from build123d import *

# Parameters (mm, degrees)
CUT_EXTRUDE1_DEPTH                   = 8
M6_CLEARANCE_HOLE1_D                 = 7
M6_CLEARANCE_HOLE1_DEPTH             = 14
M6_CLEARANCE_HOLE1_CSINK_D           = 7.05
M6_CLEARANCE_HOLE1_CSINK_ANGLE       = 90
CIRPATTERN1_COUNT                    = 4
F_6_1_6_1_DIAMETER_HOLE1_D           = 6.1
F_6_1_6_1_DIAMETER_HOLE1_DEPTH       = 14
F_6_1_6_1_DIAMETER_HOLE1_CSINK_D     = 6.15
F_6_1_6_1_DIAMETER_HOLE1_CSINK_ANGLE = 90


with BuildPart() as part:
    # Sketch1 → Revolve1 (revolve)
    with BuildSketch(Plane.XY):
        Polygon((-14, 1), (-14, 15), (-36, 15), (-36, 13), (-38, 13), (-38, 15), (-40, 15), (-40, 4), (-49, 4), (-49, 0), (-47, 0), (-47, 2), (-45, 2), (-45, 0), (-43, 0), (-43, 1), align=None)
    revolve(axis=Axis((0, 0, 0), (0, 1, 0)))

    # Sketch2 → Cut-Extrude1 (cut)
    with BuildSketch(Plane(origin=(0, 15, 0), x_dir=(1, 0, 0), z_dir=(0, 1, 0))):
        with BuildLine():
            Line((0, 3), (29, 3))
            ThreePointArc((29, 3), (32, 0), (29, -3))
            Line((29, -3), (0, -3))
            ThreePointArc((0, -3), (-3, 0), (0, 3))
        make_face()
    extrude(amount=-CUT_EXTRUDE1_DEPTH, mode=Mode.SUBTRACT)

    # M6 Clearance Hole1
    with Locations(Plane(origin=(0, 15, 0), x_dir=(1, 0, 0), z_dir=(0, 1, 0))):
        with Locations((20.506096654, 20.506096654)):
            m6_clearance_hole1 = CounterSinkHole(M6_CLEARANCE_HOLE1_D / 2, M6_CLEARANCE_HOLE1_CSINK_D / 2, depth=M6_CLEARANCE_HOLE1_DEPTH, counter_sink_angle=M6_CLEARANCE_HOLE1_CSINK_ANGLE)

    # CirPattern1: M6 Clearance Hole1 ×4 about axis
    cirpattern1_axis = Axis((0, 0, 0), (0, 1, 0))
    for i in range(1, CIRPATTERN1_COUNT):
        add(m6_clearance_hole1.rotate(cirpattern1_axis, i * 360 / CIRPATTERN1_COUNT), mode=Mode.SUBTRACT)

    # Ø6.1 (6.1) Diameter Hole1
    with Locations(Plane(origin=(0, 15, 0), x_dir=(1, 0, 0), z_dir=(0, 1, 0))):
        with Locations((-26, 0)):
            CounterSinkHole(F_6_1_6_1_DIAMETER_HOLE1_D / 2, F_6_1_6_1_DIAMETER_HOLE1_CSINK_D / 2, depth=F_6_1_6_1_DIAMETER_HOLE1_DEPTH, counter_sink_angle=F_6_1_6_1_DIAMETER_HOLE1_CSINK_ANGLE)


solid = part.part
Work out the finished part from the listing and answer in its coordinate system (mm). A direction names the side the tool comes from. Coordinates: 2 decimals unless noted, no trailing zeros. Write each loop counter-clockwise with the first axis right and the second up, starting at its lowest first coordinate (ties: lowest second). Pieces come first, ordered by that corner, then holes. Notation, with made-up numbers: M 21.25,21 L 76.25,21 A22 ccw 76.25,39 Z; hole C 67,74.5 d3. An arc over 180 degrees is marked long. Answer as CSV lines item,"result". Start each with the question number.
Item 1: A tool of negligible diameter and unlimited length cuts with its end or side. For faces 4 (the face through (-12.932, 8.098, -5.362)), 5 (the face through (8.67, 9.42, -39.05)), 6 (the face through (-44.83, 1.01, 14.12)), from which of +Z, -Z, +X, -X, +Y, -Y can it reach the whole face along a straight path? Write none if from no direction.
Item 2: Determine the mould class of faces 1 (the face through (-45.04, 2, -3.26)), 2 (the face through (-40.2, 4, 0.2)), 3 (the face through (-26.34, 1.97, 41.32)) for opening direction X: released by +X, released by -X, zero draft, split by the parting line, or undercut.
Item 3: Section C-C on y = 11.75 is taken. Write down the section's boundary in (x, z).
Item 4: Consider L1, parallel to Z at x = 0, y = 0.8; L2, parallel to Z at x = 0, y = 9.75; L3, parallel to Z at x = -33, y = 13.5. Determine where each line is inside the solid, lowest interval first.
Item 5: Flat-ended cylindrical pins translate along their axes: P1, Ø1.5, axis at y = 13.5, z = 15, coming from the +X side; P2, Ø6.5, axis at x = 23.5, y = 10.5, coming from the -Z side; P3, Ø1.5, axis at x = 30, z = 20.5, coming from the -Y side; P4, Ø5.5, axis at x = 20.51, z = 20.51, coming from the -Y side. Find the tip coordinate at first contact, or state that the pin passes through.
Checks:
1,face 4,"+Y, -Y"
1,face 5,"+Y"
1,face 6,"-Y"
2,face 1,"undercut"
2,face 2,"zero draft"
2,face 3,"split by the parting line"
3,outline,"C 0,0 d80; hole C -26,0 d6.1; hole C -20.51,-20.51 d7; hole C -20.51,20.51 d7; hole M 13.67,-3 L 29,-3 A3 ccw 29,3 L 13.67,3 A14 ccw long Z; hole C 20.51,-20.51 d7; hole C 20.51,20.51 d7"
4,L1,"z = -49 to -47, -45 to -43, 43 to 45, 47 to 49"
4,L2,"z = -40 to -14, 14 to 40"
4,L3,"z = -22.61 to -18.84, -14.39 to 14.39, 18.84 to 22.61"
5,P1,"stops at x = 37.38"
5,P2,"stops at z = -34.5"
5,P3,"stops at y = 1"
5,P4,"passes through"
